Check sheet for the modelled part. Datum: model origin and axes. Units: mm. Round coordinates to 2 decimals unless told otherwise and drop trailing zeros. Order: outer loops, then holes, each group sorted by start corner. A loop starts at its lowest first (then second) coordinate and runs counter-clockwise, first axis right, second up.
```python
from build123d import *

# Parameters (mm, degrees)
SKETCH1_R           = 12
SKETCH1_R_2         = 9.5
BOSS_EXTRUDE1_DEPTH = 16.5
SCALE1_SCALE        = 0.75
SCALE2_SCALE        = 0.85


with BuildPart() as part:
    # Sketch1 → Boss-Extrude1 (new body)
    with BuildSketch(Plane(origin=(0, 0, 0), x_dir=(0, 1, 0), z_dir=(0, 0, 1))):
        Circle(SKETCH1_R)
        Circle(SKETCH1_R_2, mode=Mode.SUBTRACT)
    extrude(amount=BOSS_EXTRUDE1_DEPTH)


with BuildPart() as part_1:
    # Scale1: scaled about (0, 0, 8.25)
    add(part.part.scale(SCALE1_SCALE).moved(Location((0, 0, 2.0625))))


with BuildPart() as part_2:
    # Scale2: scaled about (0, 0, 8.25)
    add(part_1.part.scale(SCALE2_SCALE).moved(Location((0, 0, 1.2375))))


solid = part_2.part
```
Item 1: Scan lines: line 1 along Y through (x, z) = (0, 9.25); line 2 along X through (y, z) = (-1, 10). Record each from-to range of solid material in increasing order.
Answer:
line 1: y = -7.65 to -6.06, 6.06 to 7.65
line 2: x = -7.58 to -5.97, 5.97 to 7.58
Item 2: Sectioned sample at C-C (z = 6.5). Record the cut outline in (x, y), and give its area (3 significant figures).
Answer:
outline: circle Ø15.3 at (0, 0); hole circle Ø12.11 at (0, 0)
area: 68.6 mm2
Item 3: Sectioned sample at D-D (x = 6.75). Record the cut outline in (y, z).
Answer:
outline: (-3.6, 2.99) - (3.6, 2.99) - (3.6, 13.51) - (-3.6, 13.51) - close
Item 4: Sectioned sample at A-A (y = 0). Record the cut outline in (x, z), and give its area (3 significant figures).
Answer:
outline: (-7.65, 2.99) - (-6.06, 2.99) - (-6.06, 13.51) - (-7.65, 13.51) - close; (6.06, 2.99) - (7.65, 2.99) - (7.65, 13.51) - (6.06, 13.51) - close
area: 33.5 mm2
Item 5: Go/stop test with flat-tipped pins: P1, Ø1, axis at y = 2.5, z = 10, coming from the +X side; P2, Ø5, axis at y = -5.5, z = 9.5, coming from the -X side; P3, Ø1.5, axis at y = 3.5, z = 6.5, coming from the -X side. Record where each tip stops, or that it passes through.
Answer:
P1: stops at x = 7.38
P2: stops at x = -7.04
P3: stops at x = -7.14
Item 6: Release check for a two-part mould opening along X. For faces 1 (the cylindrical face through (6.787, 3.53, 8.176)), 2 (the cylindrical face through (-1.819, 5.777, 8.176)), 3 (the flat face through (-2, 6, 13.509)) record: released by +X, released by -X, zero draft, split by the parting line, or undercut.
Answer:
face 1: split by the parting line
face 2: undercut
face 3: zero draft
